```python
from build123d import *


with BuildPart() as part:
    # Cross Section → Main (revolve)
    with BuildSketch(Plane.XY):
        with BuildLine():
            Line((-38.1, 0), (-38.1, -3.175))
            Line((-38.1, -3.175), (-41.275, -3.175))
            Line((-41.275, -3.175), (-41.275, -15.875))
            Line((-41.275, -15.875), (-44.45, -15.875))
            Line((-44.45, -15.875), (-44.45, -3.175))
            Line((-44.45, -3.175), (-51.308, -3.175))
            Line((-51.308, -3.175), (-51.308, 9.525))
            Line((-51.308, 9.525), (-49.784, 9.525))
            Line((-49.784, 9.525), (-49.784, 1.5875))
            Line((-49.784, 1.5875), (-39.6875, 1.5875))
            ThreePointArc((-39.6875, 1.5875), (-38.564967985, 1.122532015), (-38.1, 0))
        make_face()
    revolve(axis=Axis((0, 55, 0), (0, -1, 0)))


solid = part.part
```
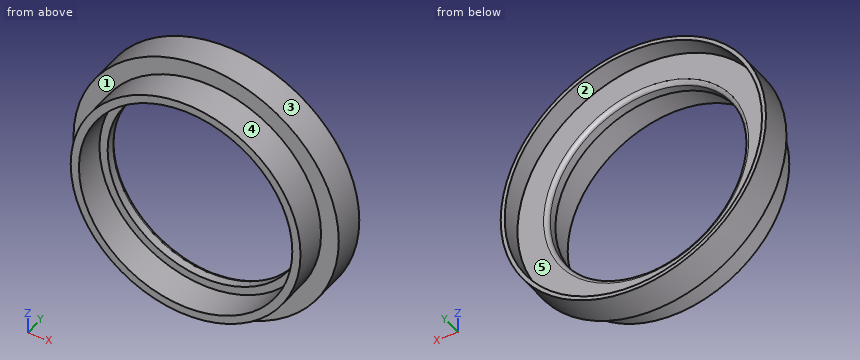
Source: CAD feature listing. Evaluate the final solid. Frame: model axes, mm. Face numbers are marked on the shaded views. A direction names the side the tool comes from. Round coordinates to 2 decimals unless told otherwise and drop trailing zeros. Loops run counter-clockwise (first coordinate to the right, second up) from the corner with the lowest first, then second, coordinate; pieces in that order, holes last.
(1) Section query C-C (y = 4.75). Output: boundary loops of the cut face in (x, z).
From the geometry:
outline: circle Ø102.62 at (0, 0); hole circle Ø99.57 at (0, 0)
(2) Pull-direction query (Z, two-part tool) for the marked faces 1, 2 and 3; classes: +Z half, -Z half, draft (parallel to the pull), parting line (faces both ways), or undercut.
From the geometry:
face 1: draft
face 2: undercut
face 3: parting line
(3) Material intervals for probe 1 along Z at (x, y) = (0, -10.75) (3 decimals); probe 2 along Z at (x, y) = (0, -2.4), sorted ascending.
From the geometry:
probe 1: z = -44.45 to -41.275, 41.275 to 44.45
probe 2: z = -51.31 to -38.1, 38.1 to 51.31
(4) Contact query for flat-ended pins moving along their axis: pin 1 Ø1 at (x, y) = (-4, -4.5) entering from +Z; pin 2 Ø12 at (x, y) = (27, 4.5) entering from -Z; pin 3 Ø5 at (x, y) = (-18.5, -11.5) entering from -Z; pin 4 Ø3 at (x, z) = (18, -31.5) entering from +Y. Output: stop coordinate, or through.
From the geometry:
pin 1: stops at z = 44.31
pin 2: stops at z = -46.81
pin 3: stops at z = -41.47
pin 4: passes through
(5) Access query for the marked faces 4 and 5. Directions: +Z, -Z, +X, -X, +Y, -Y. A direction counts if a zero-diameter tool reaches every point of the face in a straight line with its end or side. Return the directions, or none.
From the geometry:
face 4: -Y
face 5: +Y
(6) Section query D-D (y = -9). Output: boundary loops of the cut face in (x, z) (3 decimals), and give its area (3 significant figures).
From the geometry:
outline: circle Ø88.9 at (0, 0); hole circle Ø82.55 at (0, 0)
area: 855 mm2
